Source: CAD feature listing. Evaluate the final solid. Frame: model axes, mm. Face numbers are marked on the shaded views. Give positions to 0.01 mm unless a question says otherwise; leave off trailing zeros. Write each loop counter-clockwise with the first axis right and the second up, starting at its lowest first coordinate (ties: lowest second). Pieces come first, ordered by that corner, then holes. Notation, with made-up numbers: (60, -16) -> (70, -16) arc R23 ccw to (70, -1) -> close; hole circle Ø1 at (73.5, 67). An arc over 180 degrees is marked (long way). Write item = value, one per line.
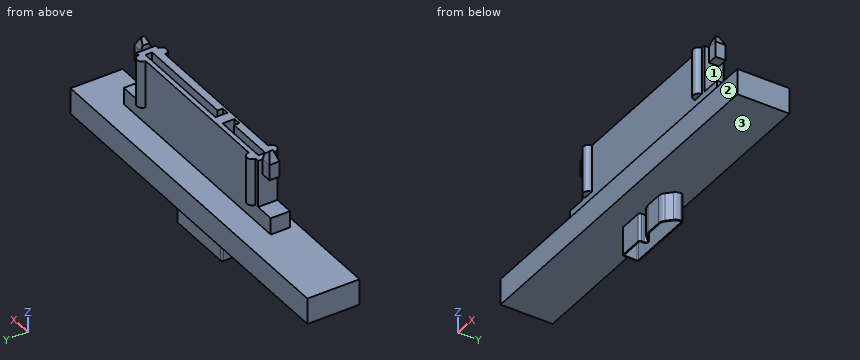
from build123d import *

# Parameters (mm, degrees)
BOSS_EXTRUDE1_DEPTH      = 2.5
BOSS_EXTRUDE1_DEPTH_BACK = 2.5
SKETCH1_W                = 70.3
SKETCH1_H                = 10
SKETCH2_W                = 43.6
SKETCH2_H                = 3.7
BOSS_EXTRUDE2_DEPTH      = 3.2
BOSS_EXTRUDE3_DEPTH      = 9.1
CUT_EXTRUDE1_DEPTH       = 10
BOSS_EXTRUDE4_DEPTH      = 0.975
BOSS_EXTRUDE4_DEPTH_BACK = 0.975
CUT_EXTRUDE2_DEPTH       = 34
CUT_EXTRUDE2_DEPTH_BACK  = 18.975
BOSS_EXTRUDE5_DEPTH      = 5.4


with BuildPart() as part:
    # Sketch1 → Boss-Extrude1 (new, two sides: drawn at the far end of the back side and taken through both)
    with BuildSketch(Plane.XY.offset(-BOSS_EXTRUDE1_DEPTH_BACK)):
        Rectangle(SKETCH1_W, SKETCH1_H)
    extrude(amount=BOSS_EXTRUDE1_DEPTH + BOSS_EXTRUDE1_DEPTH_BACK)

    # Sketch2 → Boss-Extrude2 (add)
    with BuildSketch(Plane.XY.offset(2.5)):
        with Locations((4.95, -1.65)):
            Rectangle(SKETCH2_W, SKETCH2_H)
    extrude(amount=BOSS_EXTRUDE2_DEPTH)

    # Sketch3 → Boss-Extrude3 (add)
    with BuildSketch(Plane.XY.offset(5.7)):
        with BuildLine():
            Line((-13.1, 0.2), (-12.35, 0.2))
            ThreePointArc((-12.35, 0.2), (-11.35, 1.2), (-10.35, 0.2))
            Line((-10.35, 0.2), (20.25, 0.2))
            ThreePointArc((20.25, 0.2), (21.25, 1.2), (22.25, 0.2))
            Line((22.25, 0.2), (23, 0.2))
            Line((23, 0.2), (23, -3.5))
            Line((23, -3.5), (22.25, -3.5))
            ThreePointArc((22.25, -3.5), (21.25, -4.5), (20.25, -3.5))
            Line((20.25, -3.5), (-10.35, -3.5))
            ThreePointArc((-10.35, -3.5), (-11.35, -4.5), (-12.35, -3.5))
            Line((-12.35, -3.5), (-13.1, -3.5))
            Line((-13.1, -3.5), (-13.1, 0.2))
        make_face()
    extrude(amount=BOSS_EXTRUDE3_DEPTH)

    # Sketch4 → Cut-Extrude1 (cut)
    with BuildSketch(Plane.XY.offset(14.8)):
        Polygon((-11.825, -0.7), (-1.175, -0.7), (-1.175, -3), (-2.575, -3), (-2.575, -2), (-11.825, -2), align=None)
        Polygon((0.925, -0.7), (21.725, -0.7), (21.725, -2), (2.325, -2), (2.325, -3), (0.925, -3), align=None)
    extrude(amount=-CUT_EXTRUDE1_DEPTH, mode=Mode.SUBTRACT)

    # Sketch5 → Boss-Extrude4 (add, two sides: drawn at the far end of the back side and taken through both)
    with BuildSketch(Plane(origin=(0, -1.65, 0), x_dir=(1, 0, 0), z_dir=(0, 1, 0)).offset(-BOSS_EXTRUDE4_DEPTH_BACK)):
        Polygon((-13.1, -11.8), (-15.1, -11.8), (-15.1, -14.8), (-14.1, -16.7), (-13.1, -15.75), align=None)
        Polygon((24, -16.7), (25, -14.8), (25, -11.8), (23, -11.8), (23, -15.75), align=None)
    extrude(amount=BOSS_EXTRUDE4_DEPTH + BOSS_EXTRUDE4_DEPTH_BACK)

    # Sketch6 → Cut-Extrude2 (cut, two sides: drawn at the far end of the back side and taken through both)
    with BuildSketch(Plane(origin=(0, 0, 0), x_dir=(0, 0, -1), z_dir=(1, 0, 0)).offset(-CUT_EXTRUDE2_DEPTH_BACK)):
        Polygon((-14.8, -0.675), (-16.7, -1.325), (-16.7, -0.675), align=None)
        Polygon((-14.8, -2.625), (-16.7, -2.625), (-16.7, -1.975), align=None)
    extrude(amount=CUT_EXTRUDE2_DEPTH + CUT_EXTRUDE2_DEPTH_BACK, mode=Mode.SUBTRACT)

    # Sketch7 → Boss-Extrude5 (add)
    with BuildSketch(Plane(origin=(0, 0, -2.5), x_dir=(-1, 0, 0), z_dir=(0, 0, -1))):
        with BuildLine():
            Line((-6.55, 2.9), (6.1, 2.9))
            ThreePointArc((6.1, 2.9), (6.365165043, 2.790165043), (6.475, 2.525))
            Line((6.475, 2.525), (6.475, 0.175))
            ThreePointArc((6.475, 0.175), (6.365165043, -0.090165043), (6.1, -0.2))
            Line((6.1, -0.2), (1.75, -0.2))
            ThreePointArc((1.75, -0.2), (1.484834957, -0.090165043), (1.375, 0.175))
            Line((1.375, 0.175), (1.375, 0.744669914))
            ThreePointArc((1.375, 0.744669914), (1.143506287, 1.091124739), (0.734834957, 1.009834957))
            Line((0.734834957, 1.009834957), (-0.00637085, 0.26862915))
            ThreePointArc((-0.00637085, 0.26862915), (-0.525448208, -0.078207252), (-1.1377417, -0.2))
            Line((-1.1377417, -0.2), (-4.330354687, -0.2))
            ThreePointArc((-4.330354687, -0.2), (-4.942648179, -0.078207252), (-5.461725537, 0.26862915))
            Line((-5.461725537, 0.26862915), (-6.45637085, 1.263274463))
            ThreePointArc((-6.45637085, 1.263274463), (-6.803207252, 1.782351821), (-6.925, 2.394645313))
            Line((-6.925, 2.394645313), (-6.925, 2.525))
            ThreePointArc((-6.925, 2.525), (-6.815165043, 2.790165043), (-6.55, 2.9))
        make_face()
        with BuildLine():
            Line((-5.320304181, 0.410050506), (-6.314949494, 1.404695819))
            ThreePointArc((-6.314949494, 1.404695819), (-6.618431346, 1.858888508), (-6.725, 2.394645313))
            Line((-6.725, 2.394645313), (-6.725, 2.525))
            ThreePointArc((-6.725, 2.525), (-6.673743687, 2.648743687), (-6.55, 2.7))
            Line((-6.55, 2.7), (6.1, 2.7))
            ThreePointArc((6.1, 2.7), (6.223743687, 2.648743687), (6.275, 2.525))
            Line((6.275, 2.525), (6.275, 0.175))
            ThreePointArc((6.275, 0.175), (6.223743687, 0.051256313), (6.1, 0))
            Line((6.1, 0), (1.75, 0))
            ThreePointArc((1.75, 0), (1.626256313, 0.051256313), (1.575, 0.175))
            Line((1.575, 0.175), (1.575, 0.744669914))
            ThreePointArc((1.575, 0.744669914), (1.220042974, 1.275900645), (0.593413601, 1.151256313))
            Line((0.593413601, 1.151256313), (-0.147792206, 0.410050506))
            ThreePointArc((-0.147792206, 0.410050506), (-0.601984894, 0.106568654), (-1.1377417, 0))
            Line((-1.1377417, 0), (-4.330354687, 0))
            ThreePointArc((-4.330354687, 0), (-4.866111492, 0.106568654), (-5.320304181, 0.410050506))
        make_face(mode=Mode.SUBTRACT)
    extrude(amount=BOSS_EXTRUDE5_DEPTH)


solid = part.part
1) Cut plane A-A (x = 9). Return the cut outline in (y, z), then the cut area to 3 significant figures.
Computed:
outline = (-5, -2.5) -> (5, -2.5) -> (5, 2.5) -> (0.2, 2.5) -> (0.2, 14.8) -> (-0.7, 14.8) -> (-0.7, 4.8) -> (-2, 4.8) -> (-2, 14.8) -> (-3.5, 14.8) -> (-3.5, 2.5) -> (-5, 2.5) -> close
area = 82.5 mm²
2) Material intervals for L1, parallel to X at y = -1.5, z = 8 (3 decimals); L2, parallel to X at y = 2.5, z = -3 (3 decimals); L3, parallel to Y at x = -5, z = 13, sorted ascending.
Computed:
L1 = -13.1 to -11.825, -1.175 to 0.925, 21.725 to 23
L2 = -6.475 to -6.275, 6.725 to 6.925
L3 = -3.5 to -2, -0.7 to 0.2
3) Cut plane B-B (z = 3.25). Return the cut outline in (x, y).
Computed:
outline = (-16.85, -3.5) -> (26.75, -3.5) -> (26.75, 0.2) -> (-16.85, 0.2) -> close
4) Contact query for flat-ended pins moving along their axis: pin 1 (2 mm diameter, centred on x = -14.5, z = 13.5, fed in from -Y) (3 decimals); pin 2 (6 mm diameter, centred on x = -13, y = 1.5, fed in from +Z); pin 3 (1 mm diameter, centred on x = 2, z = -5, fed in from +Y); pin 4 (4 mm diameter, centred on y = 3.5, z = 9.5, fed in from +X). Output: stop coordinate, or through.
Computed:
pin_1 = -2.625
pin_2 = 16.65
pin_3 = 2.9
pin_4 = through
5) Cut plane C-C (y = 4). Return the cut outline in (x, z).
Computed:
outline = (-35.15, -2.5) -> (35.15, -2.5) -> (35.15, 2.5) -> (-35.15, 2.5) -> close
6) Draft query along Z for the marked faces 1, 2 and 3. Return one class per face: pulls with the +Z half, pulls with the -Z half, needs draft (parallel to the pull), parting line crosses it, or undercut.
Computed:
face_1 = undercut
face_2 = needs draft
face_3 = pulls with the -Z half
